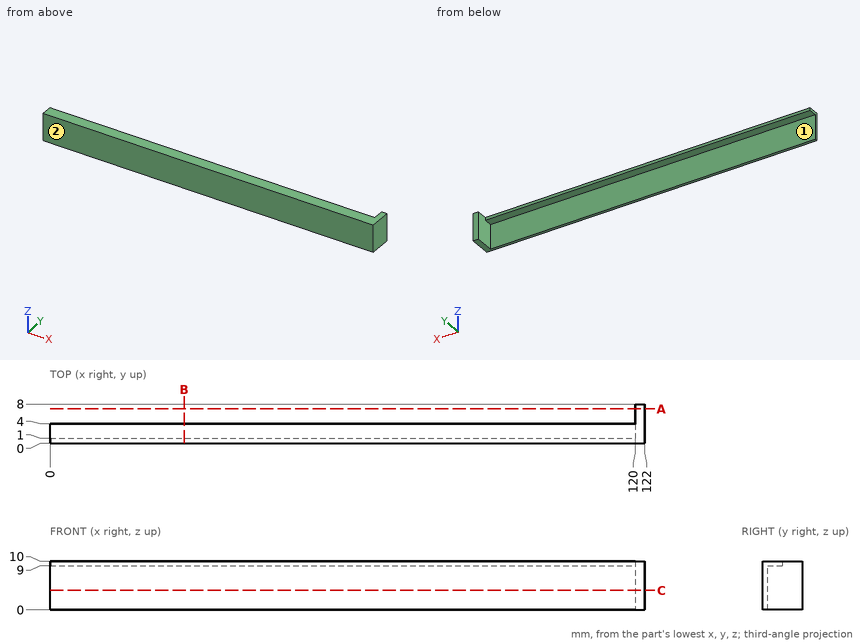
The figure shows three views and two pictorial views of one solid part (mm, origin at its lowest corner). Answer the questions. A direction names the side the tool comes from. Round coordinates to 2 decimals unless told otherwise and drop trailing zeros. Write each loop counter-clockwise with the first axis right and the second up, starting at its lowest first coordinate (ties: lowest second). Pieces come first, ordered by that corner, then holes. Notation, with made-up numbers: M 41.5,25 L 47.5,25 A20 cw 47.5,56 Z; hole C 3,3.25 d2. An arc over 180 degrees is marked long. Use a Markdown table: item, result.
1) The part is cut by section C-C on z = 4. Give the vertices of the cut face in (x, y), plus the area to 3 significant figures.
Taken from the geometry:
| item | result |
|---|---|
| outline | M 0,0 L 122,0 L 122,8 L 120,8 L 120,1 L 0,1 Z |
| area | 136 mm2 |
2) The part is cut by section A-A on y = 7. Give the vertices of the cut face in (x, z).
Taken from the geometry:
| item | result |
|---|---|
| outline | M 120,0 L 122,0 L 122,10 L 120,10 Z |
3) The part is cut by section B-B on x = 27.5. Give the vertices of the cut face in (y, z), plus the area to 3 significant figures.
Taken from the geometry:
| item | result |
|---|---|
| outline | M 0,0 L 1,0 L 1,9 L 4,9 L 4,10 L 0,10 Z |
| area | 13.0 mm2 |
4) Flat-ended cylindrical pins translate along their axes: pin 1 (2.5 mm diameter, centred on x = 90, z = 4, fed in from +Y); pin 2 (1.5 mm diameter, centred on x = 30.5, y = 2.5, fed in from -Z); pin 3 (1.1 mm diameter, centred on x = 64, z = 9.5, fed in from +Y). Find the tip coordinate at first contact, or state that the pin passes through.
Taken from the geometry:
| item | result |
|---|---|
| pin 1 | stops at y = 1 |
| pin 2 | stops at z = 9 |
| pin 3 | stops at y = 4 |
5) Consider line 1 (X direction, y = 4.25, z = 6.25); line 2 (Y direction, x = 18.5, z = 6.5); line 3 (Z direction, x = 47.5, y = 3.25). Determine where each line is inside the solid, lowest interval first. Write a range as [from, to].
Taken from the geometry:
| item | result |
|---|---|
| line 1 | x = [120, 122] |
| line 2 | y = [0, 1] |
| line 3 | z = [9, 10] |
6) Which of the six approach directions +Z, -Z, +X, -X, +Y, -Y give full straight-line access (tool end or side, diameter ignored) to the marked faces 1 and 2?
Taken from the geometry:
| item | result |
|---|---|
| face 1 | -Z, -X, +Y |
| face 2 | +Z, -Z, +X, -X, -Y |
